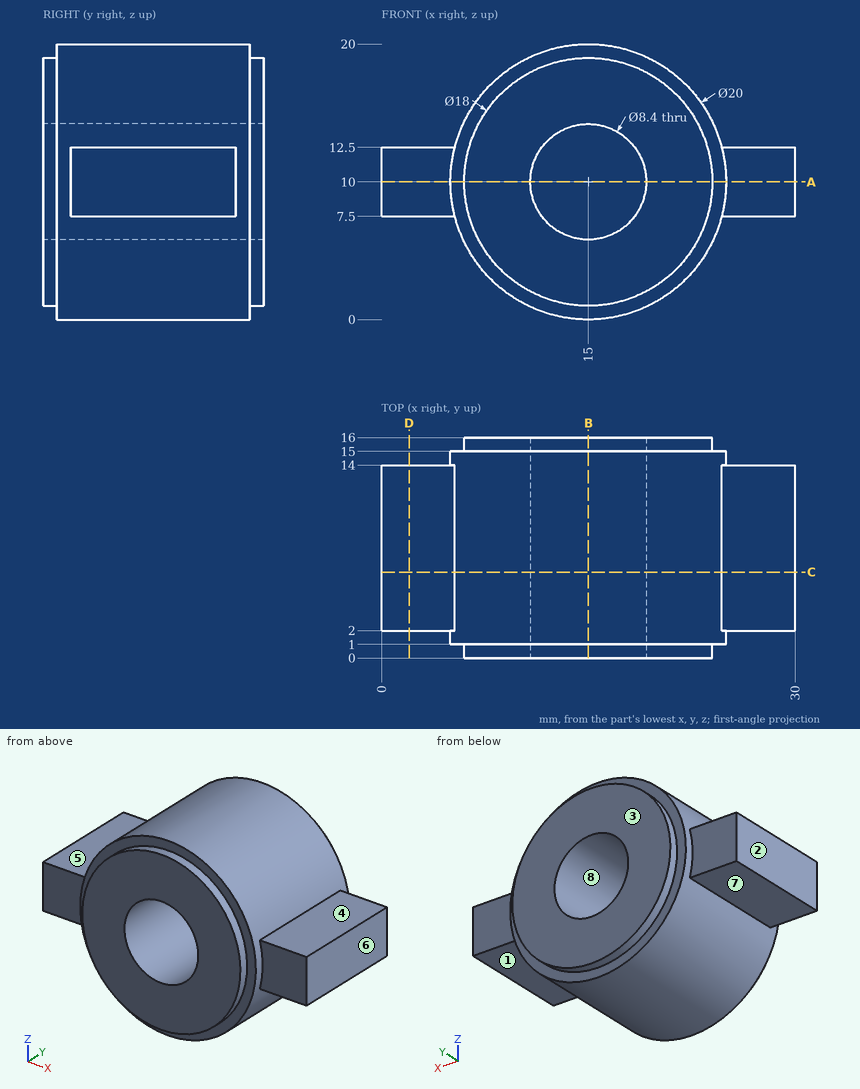
Part print with two shaded views. Sizes in mm from the minimum x, y, z corner. A direction names the side the tool comes from. Give positions to 0.01 mm unless a question says otherwise; leave off trailing zeros. Write each loop counter-clockwise with the first axis right and the second up, starting at its lowest first coordinate (ties: lowest second). Pieces come first, ordered by that corner, then holes.
1) Probe L1, parallel to X at y = 8.25, z = 10; L2, parallel to Z at x = 12.5, y = 7; L3, parallel to Z at x = 27.25, y = 7. List the from-to ranges inside material, lowest first.
Resolved:
L1: x = 0 to 10.8, 19.2 to 30
L2: z = 0.32 to 6.63, 13.37 to 19.68
L3: z = 7.5 to 12.5
2) Cut at B-B on x = 15. Write the cut outline in (y, z), then the cut area to 3 significant figures.
Resolved:
outline: (0, 1) - (1, 1) - (1, 0) - (15, 0) - (15, 1) - (16, 1) - (16, 5.8) - (0, 5.8) - close; (0, 14.2) - (16, 14.2) - (16, 19) - (15, 19) - (15, 20) - (1, 20) - (1, 19) - (0, 19) - close
area: 182 mm2
3) Cut at C-C on y = 6.25. Write the cut outline in (x, z), then the cut area to 3 significant figures.
Resolved:
outline: (0, 7.5) - (5.32, 7.5) arc R10 ccw to (24.68, 7.5) - (30, 7.5) - (30, 12.5) - (24.68, 12.5) arc R10 ccw to (5.32, 12.5) - (0, 12.5) - close; hole circle Ø8.4 at (15, 10)
area: 310 mm2
4) Pin check, flat tips, straight feed: pin 1 (4 mm diameter, centred on x = 16.5, z = 5, fed in from -Y); pin 2 (4.5 mm diameter, centred on x = 26, y = 7, fed in from +Z); pin 3 (1.5 mm diameter, centred on x = 15.5, z = 11.5, fed in from +Y); pin 4 (1.5 mm diameter, centred on x = 2, z = 11, fed in from +Y). Stop position of each tip, or through.
Resolved:
pin 1: stops at y = 0
pin 2: stops at z = 14.84
pin 3: passes through
pin 4: stops at y = 14
5) Cut at D-D on x = 2. Write the cut outline in (y, z).
Resolved:
outline: (2, 7.5) - (14, 7.5) - (14, 12.5) - (2, 12.5) - close
6) Which spindle directions (+Z, -Z, +X, -X, +Y, -Y) get a long thin tool onto all of the face, cutting with end or side? Do the marked faces 1, 2, 3, 4 and 5. Say none if no direction does.
Resolved:
face 1: -Z, +X, +Y, -Y
face 2: +Z, -Z, -X, +Y, -Y
face 3: +Z, -Z, +X, -X, +Y
face 4: +Z, +X, +Y, -Y
face 5: +Z, -X, +Y, -Y
7) Two-plate mould, pull along X, no slides. Class the marked faces 6, 7 and 8: released by +X, released by -X, zero draft, split by the parting line, or undercut.
Resolved:
face 6: released by +X
face 7: zero draft
face 8: undercut
8) Cut at A-A on z = 10. Write the cut outline in (x, y), then the cut area to 3 significant figures.
Resolved:
outline: (0, 2) - (5, 2) - (5, 1) - (6, 1) - (6, 0) - (10.8, 0) - (10.8, 16) - (6, 16) - (6, 15) - (5, 15) - (5, 14) - (0, 14) - close; (19.2, 0) - (24, 0) - (24, 1) - (25, 1) - (25, 2) - (30, 2) - (30, 14) - (25, 14) - (25, 15) - (24, 15) - (24, 16) - (19.2, 16) - close
area: 302 mm2
